Verification items for the finished model (mm, model axes). A direction names the side the tool comes from. Coordinates: 2 decimals unless noted, no trailing zeros. Write each loop counter-clockwise with the first axis right and the second up, starting at its lowest first coordinate (ties: lowest second). Pieces come first, ordered by that corner, then holes. Notation, with made-up numbers: (14, 16) -> (64, 16) arc R17 cw to (64, 22) -> close; hole circle Ø5 at (28.5, -0.5). An arc over 180 degrees is marked (long way). Answer in a Markdown table with one row per item.
```python
from build123d import *

# Parameters (mm, degrees)
SKETCH_1_W          = 45
SKETCH_1_H          = 20
EXTRUDE_1_DEPTH     = 2.5
SKETCH_3_R          = 1.55
CUT_EXTRUDE_1_DEPTH = 32.5
FILLET_1_R          = 2
SKETCH_4_W          = 21
SKETCH_4_H          = 12
CUT_EXTRUDE_2_DEPTH = 30
FILLET_2_R          = 2


with BuildPart() as part:
    # 草图1 → 凸台-拉伸1 (new body, symmetric)
    with BuildSketch(Plane.XY):
        Rectangle(SKETCH_1_W, SKETCH_1_H)
    extrude(amount=EXTRUDE_1_DEPTH, both=True)

    # 草图3 → 切除-拉伸1 (cut, symmetric)
    with BuildSketch(Plane.XY.offset(2.5)):
        with Locations((16, 5)):
            Circle(SKETCH_3_R)
        with Locations((-16, 5)):
            Circle(SKETCH_3_R)
        with Locations((-16, -5)):
            Circle(SKETCH_3_R)
        with Locations((16, -5)):
            Circle(SKETCH_3_R)
    extrude(amount=CUT_EXTRUDE_1_DEPTH, both=True, mode=Mode.SUBTRACT)

    # 圆角1
    fillet_1_edges = [part.edges().sort_by_distance(p)[0] for p in [
        (22.5, -10, 0),
        (-22.5, -10, 0),
        (-22.5, 10, 0),
        (22.5, 10, 0),
    ]]
    fillet(fillet_1_edges, radius=FILLET_1_R)

    # 草图4 → 切除-拉伸2 (cut)
    with BuildSketch(Plane.XY.offset(2.5)):
        Rectangle(SKETCH_4_W, SKETCH_4_H)
    extrude(amount=-CUT_EXTRUDE_2_DEPTH, mode=Mode.SUBTRACT)

    # 圆角2
    fillet_2_edges = [part.edges().sort_by_distance(p)[0] for p in [
        (10.5, 6, 0),
        (10.5, -6, 0),
        (-10.5, -6, 0),
        (-10.5, 6, 0),
    ]]
    fillet(fillet_2_edges, radius=FILLET_2_R)


solid = part.part
```
1. Mould release check, pull along X, two halves, no side actions. Record for faces 3 (the cylindrical face through (-21.93, -9.4, 0.04)), 4 (the cylindrical face through (-9.9, -5.43, -0.04)), 5 (the flat face through (0, 7, -2.5)), 6 (the cylindrical face through (14.45, -4.93, 0.04)): released by +X, released by -X, zero draft, split by the parting line, or undercut.
Geometry says:
| item | result |
|---|---|
| face 3 | released by -X |
| face 4 | undercut |
| face 5 | zero draft |
| face 6 | undercut |
2. Section check D-D, the plane x = 16. Record the boundary of the cut face in (y, z), plus the area to 3 significant figures.
Geometry says:
| item | result |
|---|---|
| outline | (-10, -2.5) -> (-6.55, -2.5) -> (-6.55, 2.5) -> (-10, 2.5) -> close; (-3.45, -2.5) -> (3.45, -2.5) -> (3.45, 2.5) -> (-3.45, 2.5) -> close; (6.55, -2.5) -> (10, -2.5) -> (10, 2.5) -> (6.55, 2.5) -> close |
| area | 69.0 mm^2 |
3. Tool access check on faces 1 (the flat face through (-10.5, 0, 0)), 2 (the cylindrical face through (21.9, -9.43, 0.04)). Record the directions out of +Z, -Z, +X, -X, +Y, -Y that give a thin tool (end or side, any length) a straight path to the whole face; none if there is none.
Geometry says:
| item | result |
|---|---|
| face 1 | +Z, -Z |
| face 2 | +Z, -Z, +X, -Y |
4. Thickness scan on line 1 (Y direction, x = 16, z = -0.9); line 2 (X direction, y = -3, z = 1.75); line 3 (Y direction, x = -6.5, z = -1.2). Record the ranges inside material, lowest first. Write a range as from..to.
Geometry says:
| item | result |
|---|---|
| line 1 | -10..-6.55, -3.45..3.45, 6.55..10 |
| line 2 | -22.5..-10.5, 10.5..22.5 |
| line 3 | -10..-6, 6..10 |
5. Section check B-B, the plane z = -1.9. Record the boundary of the cut face in (x, y), plus the area to 3 significant figures.
Geometry says:
| item | result |
|---|---|
| outline | (-22.5, -8) arc R2 ccw to (-20.5, -10) -> (20.5, -10) arc R2 ccw to (22.5, -8) -> (22.5, 8) arc R2 ccw to (20.5, 10) -> (-20.5, 10) arc R2 ccw to (-22.5, 8) -> close; hole circle Ø3.1 at (-16, -5); hole circle Ø3.1 at (-16, 5); hole (-10.5, -4) arc R2 ccw to (-8.5, -6) -> (8.5, -6) arc R2 ccw to (10.5, -4) -> (10.5, 4) arc R2 ccw to (8.5, 6) -> (-8.5, 6) arc R2 ccw to (-10.5, 4) -> close; hole circle Ø3.1 at (16, -5); hole circle Ø3.1 at (16, 5) |
| area | 618 mm^2 |
6. Section check A-A, the plane x = 5.5. Record the boundary of the cut face in (y, z).
Geometry says:
| item | result |
|---|---|
| outline | (-10, -2.5) -> (-6, -2.5) -> (-6, 2.5) -> (-10, 2.5) -> close; (6, -2.5) -> (10, -2.5) -> (10, 2.5) -> (6, 2.5) -> close |
7. Section check C-C, the plane y = 0. Record the boundary of the cut face in (x, z).
Geometry says:
| item | result |
|---|---|
| outline | (-22.5, -2.5) -> (-10.5, -2.5) -> (-10.5, 2.5) -> (-22.5, 2.5) -> close; (10.5, -2.5) -> (22.5, -2.5) -> (22.5, 2.5) -> (10.5, 2.5) -> close |
